Drawing for the job (mm, zero at the part's lowest x, y, z). A direction names the side the tool comes from. Coordinates: 2 decimals unless noted, no trailing zeros. Order: outer loops, then holes, each group sorted by start corner. A loop starts at its lowest first (then second) coordinate and runs counter-clockwise, first axis right, second up. Notation, with made-up numbers: M 22.5,-38.5 L 28.5,-38.5 A38 cw 28.5,0.5 Z; hole C 89.25,87 d1. An arc over 180 degrees is marked long. Write item = value, one per line. Start each with the question number.
Q1. Band-saw the part on A-A on x = 11.5. Write the cut outline in (y, z).
Q2. Drill centre lines: probe 1 along Z at (x, y) = (11.5, 0.65); probe 2 along Y at (x, z) = (4.75, 9); probe 3 along X at (y, z) = (9, 11.25). Where is each one in solid material? Low to high.
Q3. Pin check, flat tips, straight feed: P1, Ø6, axis at x = 6, z = 7.5, coming from the -Y side; P2, Ø1, axis at x = 3.5, y = 8.5, coming from the -Z side. Stop position of each tip, or through.
Q4. Band-saw the part on C-C on z = 6. Write the cut outline in (x, y), plus the area to 3 significant figures.
Q5. 3-axis set-ups, long thin cutter, end or side, ignore diameter. For the marked faces 4 and 5: which of +Z, -Z, +X, -X, +Y, -Y reach the whole face in a straight line?
Q6. Pull direction Z, two halves, no side cores. Call the marked faces 1, 2 and 3: released by +Z, released by -Z, zero draft, split by the parting line, or undercut.
Q7. Band-saw the part on D-D on x = 10. Write the cut outline in (y, z).
Q8. Band-saw the part on B-B on x = 7. Write the cut outline in (y, z).
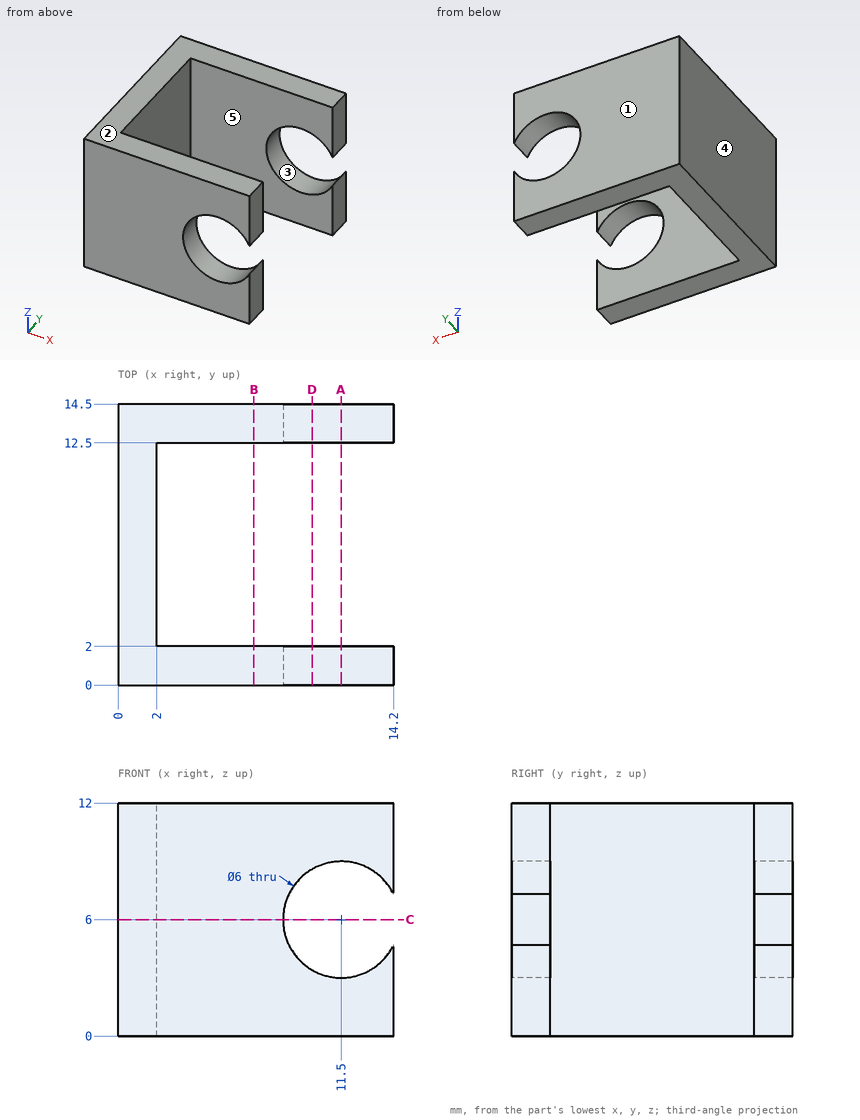
Recorded:
q1.outline = M 0,0 L 2,0 L 2,3 L 0,3 Z; M 0,9 L 2,9 L 2,12 L 0,12 Z; M 12.5,0 L 14.5,0 L 14.5,3 L 12.5,3 Z; M 12.5,9 L 14.5,9 L 14.5,12 L 12.5,12 Z
q2.probe_1 = 0 to 3, 9 to 12
q2.probe_2 = 0 to 2, 12.5 to 14.5
q2.probe_3 = 0 to 2
q3.P1 = 0
q3.P2 = through
q4.outline = M 0,0 L 8.5,0 L 8.5,2 L 2,2 L 2,12.5 L 8.5,12.5 L 8.5,14.5 L 0,14.5 Z
q4.area = 55.0 mm2
q5.face_4 = +Z, -Z, -X, +Y, -Y
q5.face_5 = +Z, -Z, +X
q6.face_1 = zero draft
q6.face_2 = released by +Z
q6.face_3 = undercut
q7.outline = M 0,0 L 2,0 L 2,3.4 L 0,3.4 Z; M 0,8.6 L 2,8.6 L 2,12 L 0,12 Z; M 12.5,0 L 14.5,0 L 14.5,3.4 L 12.5,3.4 Z; M 12.5,8.6 L 14.5,8.6 L 14.5,12 L 12.5,12 Z
q8.outline = M 0,0 L 2,0 L 2,12 L 0,12 Z; M 12.5,0 L 14.5,0 L 14.5,12 L 12.5,12 Z
